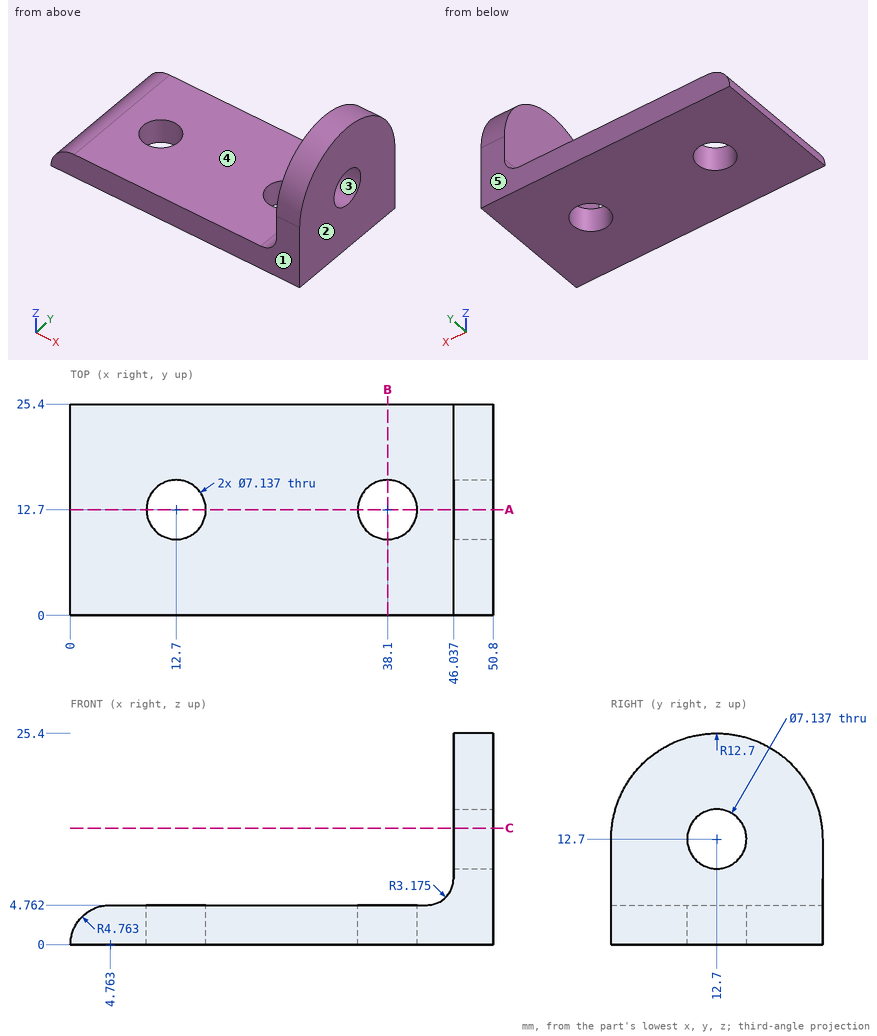
Could you check a few things on this drawing? It's one solid part, dimensions in mm from its lowest x, y, z. A direction names the side the tool comes from. Give positions to 0.01 mm unless a question says otherwise; leave off trailing zeros. Order: outer loops, then holes, each group sorted by start corner. A loop starts at its lowest first (then second) coordinate and runs counter-clockwise, first axis right, second up.
1. For pin 1 (2 mm diameter, centred on x = 40.5, y = 17, fed in from +Z); pin 2 (8.5 mm diameter, centred on y = 14, z = 19, fed in from -X), each with a flat end and sliding along its axis, tell me the tip position at first contact or that it passes through.
Answers below:
pin 1: stops at z = 4.76
pin 2: stops at x = 46.04
2. Suppose I cut it at A-A (y = 12.7). State how many separate pieces and enclosed holes the cut face has.
Answers below:
separate pieces: 4
enclosed holes: 0
3. I need wall thicknesses on L1, parallel to Y at x = 47.05, z = 12.7; L2, parallel to Z at x = 43, y = 8.5 (1 decimal); L3, parallel to X at y = 6.25, z = 10. Which ranges of each line are inside material? Lowest first, please.
Answers below:
L1: y = 0 to 9.13, 16.27 to 25.4
L2: z = 0 to 4.8
L3: x = 46.04 to 50.8
4. Which directions (+Z, -Z, +X, -X, +Y, -Y) give clear straight access to the entire face, cutting with the end or side of a thin tool? Please do the marked faces 4 and 5.
Answers below:
face 4: +Z, -X, +Y, -Y
face 5: +Z, -Z, +X, -X, +Y
5. Suppose I cut it at B-B (x = 38.1). Write out the boundary of the cut face in (y, z).
Answers below:
outline: (0, 0) - (9.13, 0) - (9.13, 4.76) - (0, 4.76) - close; (16.27, 0) - (25.4, 0) - (25.4, 4.76) - (16.27, 4.76) - close
6. Suppose I cut it at C-C (z = 14). Write out the boundary of the cut face in (x, y).
Answers below:
outline: (46.04, 0.07) - (50.8, 0.07) - (50.8, 9.38) - (46.04, 9.38) - close; (46.04, 16.02) - (50.8, 16.02) - (50.8, 25.33) - (46.04, 25.33) - close
7. Thinking about a two-plate mould opening in Y: for the marked faces 1, 2 and 3, which applies, +Y half, -Y half, draft (parallel to the pull), parting line (faces both ways), or undercut?
Answers below:
face 1: -Y half
face 2: draft
face 3: undercut
